The listing builds one solid part. Answer for the finished solid, in the listing's coordinates (mm). Face numbers are marked on the shaded views. A direction names the side the tool comes from. Give positions to 0.01 mm unless a question says otherwise; leave off trailing zeros. Write each loop counter-clockwise with the first axis right and the second up, starting at its lowest first coordinate (ties: lowest second). Pieces come first, ordered by that corner, then holes. Notation, with made-up numbers: (-38, -31.5) - (10, -31.5) arc R24 ccw to (10, -9.5) - close; hole circle Ø6 at (-16, -36.5). An arc over 180 degrees is marked (long way). Return JSON: item names as keys, results as strings.
from build123d import *

# Parameters (mm, degrees)
SKETCH_W     = 34
SKETCH_H     = 34
PAD_DEPTH    = 20
POCKET_DEPTH = 20


with BuildPart() as part:
    # Sketch → Pad (new body)
    with BuildSketch(Plane.XY):
        with Locations((17, 17)):
            Rectangle(SKETCH_W, SKETCH_H)
    extrude(amount=PAD_DEPTH)

    # Sketch001 (on Face6 of Pad) → Pocket (cut)
    with BuildSketch(Plane.XY.offset(20)):
        Polygon((6.5, 27.5), (14, 27.5), (14, 23.5), (17, 21.5), (20, 23.5), (20, 27.5), (27.5, 27.5), (27.5, 19.5), (23.5, 19.5), (21.5, 17), (23.5, 14), (27.5, 14), (27.5, 6.5), (20, 6.5), (20, 10.5), (17, 12.5), (14, 10.5), (14, 6.5), (6.5, 6.5), (6.5, 14), (10.5, 14), (12.5, 17), (10.5, 19.5), (6.5, 19.5), align=None)
    extrude(amount=-POCKET_DEPTH, mode=Mode.SUBTRACT)


solid = part.part
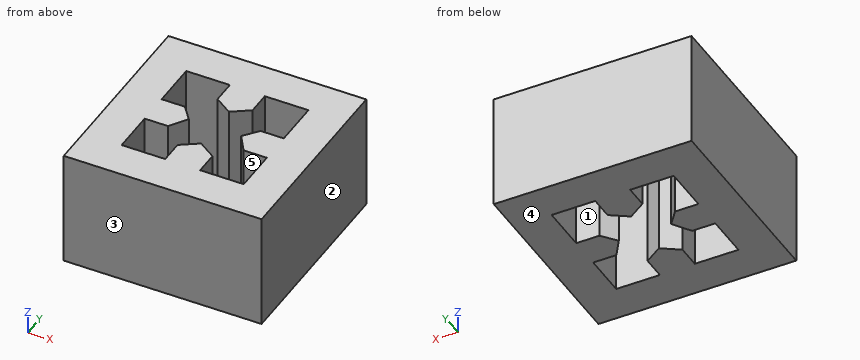
Item 1: A cutting plane is placed at A-A on x = 20.5. Determine the outline of the cut face in (y, z), then the cut area to 3 significant figures.
Answer below:
{"outline": "(0, 0) - (6.5, 0) - (6.5, 20) - (0, 20) - close; (27.5, 0) - (34, 0) - (34, 20) - (27.5, 20) - close", "area": "260 mm²"}
Item 2: For the marked faces 4 and 5, determine the directions among +Z, -Z, +X, -X, +Y, -Y from which every point of the face is accessible in a straight line to the end or side of a thin tool.
Answer below:
{"face 4": "-Z, +X, -X, +Y, -Y", "face 5": "+Z, -Z"}
Item 3: A cutting plane is placed at C-C on z = 2. Determine the outline of the cut face in (x, y).
Answer below:
{"outline": "(0, 0) - (34, 0) - (34, 34) - (0, 34) - close; hole (6.5, 6.5) - (14, 6.5) - (14, 10.5) - (17, 12.5) - (20, 10.5) - (20, 6.5) - (27.5, 6.5) - (27.5, 14) - (23.5, 14) - (21.5, 17) - (23.5, 19.5) - (27.5, 19.5) - (27.5, 27.5) - (20, 27.5) - (20, 23.5) - (17, 21.5) - (14, 23.5) - (14, 27.5) - (6.5, 27.5) - (6.5, 19.5) - (10.5, 19.5) - (12.5, 17) - (10.5, 14) - (6.5, 14) - close"}
Item 4: A cutting plane is placed at D-D on y = 18.5. Determine the outline of the cut face in (x, z).
Answer below:
{"outline": "(0, 0) - (11.3, 0) - (11.3, 20) - (0, 20) - close; (22.7, 0) - (34, 0) - (34, 20) - (22.7, 20) - close"}
Item 5: The mould has two halves that part along X. Classify the marked faces 1, 2 and 3: +X half, -X half, draft (parallel to the pull), parting line (faces both ways), or undercut.
Answer below:
{"face 1": "undercut", "face 2": "+X half", "face 3": "draft"}
Item 6: A cutting plane is placed at B-B on y = 12. Determine the outline of the cut face in (x, z), then the cut area to 3 significant figures.
Answer below:
{"outline": "(0, 0) - (6.5, 0) - (6.5, 20) - (0, 20) - close; (16.25, 0) - (17.75, 0) - (17.75, 20) - (16.25, 20) - close; (27.5, 0) - (34, 0) - (34, 20) - (27.5, 20) - close", "area": "290 mm²"}
Item 7: Consider L1, parallel to Y at x = 24.5, z = 16.75; L2, parallel to X at y = 7, z = 13.5; L3, parallel to Y at x = 17, z = 7.5. Determine where each line is inside the solid, lowest interval first.
Answer below:
{"L1": "y = 0 to 6.5, 14 to 19.5, 27.5 to 34", "L2": "x = 0 to 6.5, 14 to 20, 27.5 to 34", "L3": "y = 0 to 12.5, 21.5 to 34"}
